```python
from build123d import *

# Parameters (mm, degrees)
SKETCH1_R           = 57.5
SKETCH1_R_2         = 1.75
SKETCH1_R_3         = 26
SKETCH1_R_4         = 2.5
BOSS_EXTRUDE1_DEPTH = 7


with BuildPart() as part:
    # Sketch1 → Boss-Extrude1 (new body)
    with BuildSketch(Plane(origin=(0, 0, 0), x_dir=(1, 0, 0), z_dir=(0, 1, 0))):
        with Locations(Location((0, 0, 0), (0, 0, 270))):
            Circle(SKETCH1_R)
        with Locations(Location((0, 54, 0), (0, 0, 270))):
            Circle(SKETCH1_R_2, mode=Mode.SUBTRACT)
        with Locations(Location((27, 46.765371804, 0), (0, 0, 270))):
            Circle(SKETCH1_R_2, mode=Mode.SUBTRACT)
        with Locations(Location((46.765371804, 27, 0), (0, 0, 270))):
            Circle(SKETCH1_R_2, mode=Mode.SUBTRACT)
        with Locations(Location((54, 0, 0), (0, 0, 270))):
            Circle(SKETCH1_R_2, mode=Mode.SUBTRACT)
        with Locations(Location((46.765371804, -27, 0), (0, 0, 270))):
            Circle(SKETCH1_R_2, mode=Mode.SUBTRACT)
        with Locations(Location((27, -46.765371804, 0), (0, 0, 270))):
            Circle(SKETCH1_R_2, mode=Mode.SUBTRACT)
        with Locations(Location((0, -54, 0), (0, 0, 270))):
            Circle(SKETCH1_R_2, mode=Mode.SUBTRACT)
        with Locations(Location((-27, -46.765371804, 0), (0, 0, 270))):
            Circle(SKETCH1_R_2, mode=Mode.SUBTRACT)
        with Locations(Location((-46.765371804, -27, 0), (0, 0, 270))):
            Circle(SKETCH1_R_2, mode=Mode.SUBTRACT)
        with Locations(Location((-54, 0, 0), (0, 0, 270))):
            Circle(SKETCH1_R_2, mode=Mode.SUBTRACT)
        with Locations(Location((-46.765371804, 27, 0), (0, 0, 270))):
            Circle(SKETCH1_R_2, mode=Mode.SUBTRACT)
        with Locations(Location((-27, 46.765371804, 0), (0, 0, 270))):
            Circle(SKETCH1_R_2, mode=Mode.SUBTRACT)
        with Locations(Location((0, 0, 0), (0, 0, 270))):
            Circle(SKETCH1_R_3, mode=Mode.SUBTRACT)
        with Locations(Location((0, 45, 0), (0, 0, 270))):
            Circle(SKETCH1_R_4, mode=Mode.SUBTRACT)
        with Locations(Location((24.328836786, 37.856408977, 0), (0, 0, 270))):
            Circle(SKETCH1_R_4, mode=Mode.SUBTRACT)
        with Locations(Location((40.933439791, 18.693675585, 0), (0, 0, 270))):
            Circle(SKETCH1_R_4, mode=Mode.SUBTRACT)
        with Locations(Location((44.541964885, -6.404167722, 0), (0, 0, 270))):
            Circle(SKETCH1_R_4, mode=Mode.SUBTRACT)
        with Locations(Location((34.008730846, -29.468733028, 0), (0, 0, 270))):
            Circle(SKETCH1_R_4, mode=Mode.SUBTRACT)
        with Locations(Location((12.677965058, -43.177183813, 0), (0, 0, 270))):
            Circle(SKETCH1_R_4, mode=Mode.SUBTRACT)
        with Locations(Location((-12.677965058, -43.177183813, 0), (0, 0, 270))):
            Circle(SKETCH1_R_4, mode=Mode.SUBTRACT)
        with Locations(Location((-34.008730846, -29.468733028, 0), (0, 0, 270))):
            Circle(SKETCH1_R_4, mode=Mode.SUBTRACT)
        with Locations(Location((-44.541964885, -6.404167722, 0), (0, 0, 270))):
            Circle(SKETCH1_R_4, mode=Mode.SUBTRACT)
        with Locations(Location((-40.933439791, 18.693675585, 0), (0, 0, 270))):
            Circle(SKETCH1_R_4, mode=Mode.SUBTRACT)
        with Locations(Location((-24.328836786, 37.856408977, 0), (0, 0, 270))):
            Circle(SKETCH1_R_4, mode=Mode.SUBTRACT)
    extrude(amount=BOSS_EXTRUDE1_DEPTH)


solid = part.part
```
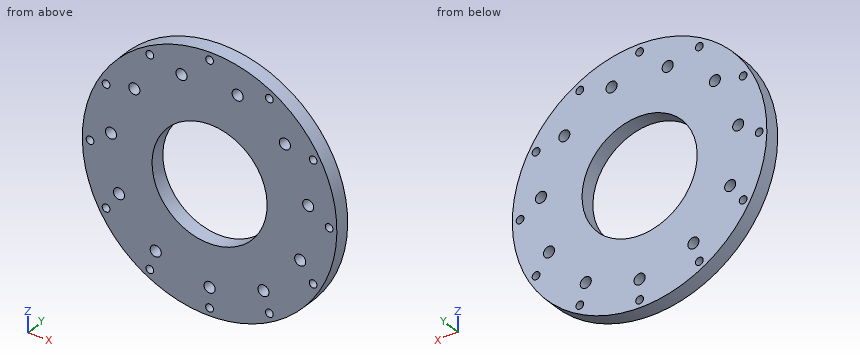
Here's how the part is built. I have some questions about the finished solid (model axes, mm). Give positions to 0.01 mm unless a question says otherwise; leave off trailing zeros. Order: outer loops, then holes, each group sorted by start corner. A loop starts at its lowest first (then second) coordinate and runs counter-clockwise, first axis right, second up. Notation, with made-up numbers: M 78,73 L 132,73 A30 cw 132,102 Z; hole C 62,56.25 d5. An arc over 180 degrees is marked long. Use a Markdown table: item, result. Add a question column.
1. Suppose I cut it at D-D (y = 5). Give the number of separate pieces and of enclosed holes in the cut face, and give its area (3 significant figures).
2. I need wall thicknesses on probe 1 along Z at (x, y) = (12, 2.75); probe 2 along X at (y, z) = (6.5, 47); probe 3 along Z at (x, y) = (-42.5, 3.25). Which ranges of each line are inside material? Lowest first, please. Write a range as from..to.
3. For pin 1 Ø4 at (x, z) = (-46.77, 27) entering from -Y; pin 2 Ø4 at (y, z) = (2.5, 20.5) entering from +X; pin 3 Ø4 at (y, z) = (2.5, -44) entering from -X; pin 4 Ø2 at (x, y) = (-30.5, 5) entering from +Z, each with a flat end and sliding along its axis, tell me the tip position at first contact or that it passes through.
4. Suppose I cut it at A-A (x = 0). List the corners of the cut face in (y, z) for me, and give its area (3 significant figures).
5. Suppose I cut it at B-B (z = 20). List the corners of the cut face in (x, y) for me, and give its area (3 significant figures).
6. Suppose I cut it at C-C (z = 0). List the corners of the cut face in (x, y) for me, and give its area (3 significant figures).
Results list:
| question | item | result |
|---|---|---|
| 1 | separate pieces | 1 |
| 1 | enclosed holes | 24 |
| 1 | area | 7,930 mm² |
| 2 | probe 1 | z = -56.23..-23.07, 23.07..40.77, 45.58..56.23 |
| 2 | probe 2 | x = -33.12..-28.73, -25.27..25.27, 28.73..33.12 |
| 2 | probe 3 | z = -38.73..-20.64, -16.75..4.96, 7.85..38.73 |
| 3 | pin 1 | stops at y = 0 |
| 3 | pin 2 | stops at x = 54.44 |
| 3 | pin 3 | stops at x = -39.27 |
| 3 | pin 4 | stops at z = 49.36 |
| 4 | outline | M 0,-57.5 L 7,-57.5 L 7,-55.75 L 0,-55.75 Z; M 0,-52.25 L 7,-52.25 L 7,-47.5 L 0,-47.5 Z; M 0,-42.5 L 7,-42.5 L 7,-26 L 0,-26 Z; M 0,26 L 7,26 L 7,52.25 L 0,52.25 Z; M 0,55.75 L 7,55.75 L 7,57.5 L 0,57.5 Z |
| 4 | area | 357 mm² |
| 5 | outline | M -53.91,0 L -16.61,0 L -16.61,7 L -53.91,7 Z; M 16.61,0 L 53.91,0 L 53.91,7 L 16.61,7 Z |
| 5 | area | 522 mm² |
| 6 | outline | M -57.5,0 L -55.75,0 L -55.75,7 L -57.5,7 Z; M -52.25,0 L -26,0 L -26,7 L -52.25,7 Z; M 26,0 L 52.25,0 L 52.25,7 L 26,7 Z; M 55.75,0 L 57.5,0 L 57.5,7 L 55.75,7 Z |
| 6 | area | 392 mm² |
